from build123d import *

# Parameters (mm, degrees)
SKETCH1_R               = 1.5
BASE_EXTRUDE_DEPTH      = 5
BASE_EXTRUDE_DEPTH_BACK = 0.0001
CUT_EXTRUDE1_DEPTH      = 1.799999969
CUT_EXTRUDE1_TAPER      = 2


with BuildPart() as part:
    # Sketch1 → Base-Extrude (new body, two sides)
    with BuildSketch(Plane.XY) as base_extrude_sk:
        Circle(SKETCH1_R)
    extrude(amount=BASE_EXTRUDE_DEPTH)
    extrude(base_extrude_sk.sketch, amount=-BASE_EXTRUDE_DEPTH_BACK)

    # Sketch6 → Boss-Revolve2 (revolve)
    with BuildSketch(Plane(origin=(0, 0, 0), x_dir=(1, 0, 0), z_dir=(0, 1, 0))):
        with BuildLine():
            Line((0, -5), (2.7999999, -5))
            Line((2.7999999, -5), (2.7999999, -6.54246308))
            ThreePointArc((2.7999999, -6.54246308), (1.46418655, -7.180811406), (0, -7.4))
            Line((0, -7.4), (0, -5))
        make_face()
    revolve(axis=Axis((0, 0, -0.393620135), (0, 0, 1)))

    # Sketch7 → Cut-Extrude1 (cut)
    with BuildSketch(Plane(origin=(0, 0, 7.7000001), x_dir=(-1, 0, 0), z_dir=(0, 0, -1))):
        with BuildLine():
            ThreePointArc((0.205000004, 1.48592565), (0, 1.500000013), (-0.205000004, 1.48592565))
            Line((-0.205000004, 1.48592565), (-0.205000004, 0.708178558))
            ThreePointArc((-0.205000004, 0.708178558), (-0.35072876, 0.355344481), (-0.702967546, 0.208182689))
            Line((-0.702967546, 0.208182689), (-1.48592565, 0.205000004))
            ThreePointArc((-1.48592565, 0.205000004), (-1.500000013, 0), (-1.48592565, -0.205000004))
            Line((-1.48592565, -0.205000004), (-0.702967546, -0.208182689))
            ThreePointArc((-0.702967546, -0.208182689), (-0.35072876, -0.355344481), (-0.205000004, -0.708178558))
            Line((-0.205000004, -0.708178558), (-0.205000004, -1.48592565))
            ThreePointArc((-0.205000004, -1.48592565), (0, -1.500000013), (0.205000004, -1.48592565))
            Line((0.205000004, -1.48592565), (0.205000004, -0.708178558))
            ThreePointArc((0.205000004, -0.708178558), (0.35072876, -0.355344481), (0.702967546, -0.208182689))
            Line((0.702967546, -0.208182689), (1.48592565, -0.205000004))
            ThreePointArc((1.48592565, -0.205000004), (1.500000013, 0), (1.48592565, 0.205000004))
            Line((1.48592565, 0.205000004), (0.702967546, 0.208182689))
            ThreePointArc((0.702967546, 0.208182689), (0.35072876, 0.355344481), (0.205000004, 0.708178558))
            Line((0.205000004, 0.708178558), (0.205000004, 1.48592565))
        make_face()
    extrude(amount=CUT_EXTRUDE1_DEPTH, taper=CUT_EXTRUDE1_TAPER, mode=Mode.SUBTRACT)


solid = part.part
Check sheet for the modelled part. Datum: model origin and axes. Units: mm. Coordinates: 2 decimals unless noted, no trailing zeros. Loops run counter-clockwise (first coordinate to the right, second up) from the corner with the lowest first, then second, coordinate; pieces in that order, holes last. Notation, with made-up numbers: (31.5, 87) -> (63.5, 87) arc R27 cw to (63.5, 125) -> close; hole circle Ø9 at (84.25, 28.25). An arc over 180 degrees is marked (long way). Write item = value, one per line. Start each with the question number.
1. Section check C-C on y = 2.15. Record the cut outline in (x, z), then the cut area to 3 significant figures.
2. Draft check along X on faces 1 (the cylindrical face through (-0.607, -2.733, 5.782)), 2 (the flat face through (0, 0, 5.9)), 3 (the flat face through (0, 0, 0)). Enter one of: released by +X, released by -X, zero draft, split by the parting line, or undercut.
3. Material ranges on line 1 (Y direction, x = -0.45, z = 2); line 2 (X direction, y = -0.1, z = 6.5); line 3 (Y direction, x = 0, z = 1), recorded low to high.
4. Section check B-B on x = 2.55. Record the cut outline in (y, z), then the cut area to 3 significant figures.
5. Section check D-D on z = 5.5. Record the cut outline in (x, y), then the cut area to 3 significant figures.
6. Depth check by flat-ended pin: P1, Ø2, axis at y = 1.5, z = 5, coming from the -X side (3 decimals); P2, Ø2, axis at x = -1.5, z = 1.5, coming from the -Y side. Enter the tip coordinate at first touch or a pass-through.
7. Section check A-A on z = 0.75. Record the cut outline in (x, y).
Responses:
q1.outline = (-1.79, 5) -> (1.79, 5) -> (1.79, 6.54) arc R4.51 ccw to (-1.79, 6.54) -> close
q1.area = 6.43 mm2
q2.face_1 = split by the parting line
q2.face_2 = undercut
q2.face_3 = zero draft
q3.line_1 = -1.43 to 1.43
q3.line_2 = -2.8 to -1.45, 1.45 to 2.8
q3.line_3 = -1.5 to 1.5
q4.outline = (-1.16, 5) -> (1.16, 5) -> (1.16, 6.54) arc R4.3 ccw to (-1.16, 6.54) -> close
q4.area = 3.81 mm2
q5.outline = circle Ø5.6 at (0, 0)
q5.area = 24.6 mm2
q6.P1 = -2.755
q6.P2 = -1.41
q7.outline = circle Ø3 at (0, 0)
